from build123d import *

# Parameters (mm, degrees)
SKETCH1_R               = 129.43
BOSS_EXTRUDE1_DEPTH     = 3
CUT_EXTRUDE2_START      = -3
CUT_EXTRUDE2_DEPTH      = 4
CIRPATTERN1_COUNT       = 8
SKETCH4_R               = 3.5
SKETCH4_W               = 25
SKETCH4_H               = 25
CUT_EXTRUDE3_DEPTH      = 3
CUT_EXTRUDE4_DEPTH      = 10
CUT_EXTRUDE5_DEPTH      = 1
CUT_EXTRUDE5_DEPTH_BACK = 3
CUT_EXTRUDE6_DEPTH      = 1
CUT_EXTRUDE6_DEPTH_BACK = 3


with BuildPart() as part:
    # Sketch1 → Boss-Extrude1 (new body)
    with BuildSketch(Plane(origin=(0, 0, 0), x_dir=(1, 0, 0), z_dir=(0, 1, 0))):
        Circle(SKETCH1_R)
    extrude(amount=BOSS_EXTRUDE1_DEPTH)

    # Sketch2 → Cut-Extrude2 (cut)
    with BuildSketch(Plane(origin=(0, 3, 0), x_dir=(1, 0, 0), z_dir=(0, 1, 0)).offset(CUT_EXTRUDE2_START)):
        Polygon((-1.5, 719.582197244), (-1.5, 129.421307751), (-1.5, 119.421307751), (1.5, 119.421307751), (1.5, 129.421307751), (1.5, 719.582197244), (1.5, 1899.903976231), (-1.5, 1899.903976231), align=None)
    cut_extrude2 = extrude(amount=CUT_EXTRUDE2_DEPTH, mode=Mode.SUBTRACT)

    # CirPattern1: Cut-Extrude2 ×8 about axis
    cirpattern1_axis = Axis((0, 0, 0), (0, -1, 0))
    for i in range(1, CIRPATTERN1_COUNT):
        add(cut_extrude2.rotate(cirpattern1_axis, i * 360 / CIRPATTERN1_COUNT), mode=Mode.SUBTRACT)

    # Sketch4 → Cut-Extrude3 (cut)
    with BuildSketch(Plane(origin=(0, 3, 0), x_dir=(1, 0, 0), z_dir=(0, 1, 0))):
        with Locations((20, 20)):
            Circle(SKETCH4_R)
        with Locations((20, -20)):
            Circle(SKETCH4_R)
        with Locations((-20, -20)):
            Circle(SKETCH4_R)
        with Locations((-20, 20)):
            Circle(SKETCH4_R)
        Rectangle(SKETCH4_W, SKETCH4_H)
    extrude(amount=-CUT_EXTRUDE3_DEPTH, mode=Mode.SUBTRACT)

    # Sketch5 → Cut-Extrude4 (cut)
    with BuildSketch(Plane(origin=(0, 3, 0), x_dir=(1, 0, 0), z_dir=(0, 1, 0))):
        Polygon((-42.767689854, -111.089714666), (-39.996051256, -112.237764963), (-26.219447691, -78.978101793), (-28.991086289, -77.830051496), align=None)
        Polygon((-26.137858269, -117.978016449), (-23.366219671, -119.126066746), (-9.589616106, -85.866403575), (-12.361254704, -84.718353278), align=None)
        Polygon((53.935833667, 67.497598822), (67.712437232, 100.757261992), (64.940798634, 101.905312289), (51.164195069, 68.645649119), align=None)
        Polygon((37.306002081, 74.385900604), (51.082605647, 107.645563775), (48.310967049, 108.793614072), (34.534363484, 75.533950901), align=None)
    extrude(amount=-CUT_EXTRUDE4_DEPTH, mode=Mode.SUBTRACT)

    # Sketch6 → Cut-Extrude5 (cut, two sides)
    with BuildSketch(Plane(origin=(0, 3, 0), x_dir=(1, 0, 0), z_dir=(0, 1, 0))) as cut_extrude5_sk:
        Polygon((264.658286272, 696.415643975), (28.490193223, 126.255430735), (21.127814063, 108.481075117), (30.356179145, 104.658561141), (38.225405343, 123.656553754), (274.393498392, 693.816766994), (592.742329798, 1886.329311701), (583.007117678, 1888.928188682), align=None)
    extrude(amount=CUT_EXTRUDE5_DEPTH, mode=Mode.SUBTRACT)
    extrude(cut_extrude5_sk.sketch, amount=-CUT_EXTRUDE5_DEPTH_BACK, mode=Mode.SUBTRACT)

    # Sketch8 → Cut-Extrude6 (cut, two sides)
    with BuildSketch(Plane(origin=(0, 3, 0), x_dir=(1, 0, 0), z_dir=(0, 1, 0))) as cut_extrude6_sk:
        Polygon((-310.659690478, -692.568815319), (-69.116017705, -109.430804605), (-61.752527909, -91.653767674), (-52.555273509, -95.463395183), (-60.423899034, -114.459937644), (-301.967571807, -697.597948358), (-934.16352501, -1790.255908717), (-942.855643681, -1785.226775678), align=None)
    extrude(amount=CUT_EXTRUDE6_DEPTH, mode=Mode.SUBTRACT)
    extrude(cut_extrude6_sk.sketch, amount=-CUT_EXTRUDE6_DEPTH_BACK, mode=Mode.SUBTRACT)


solid = part.part
Model file for the job. Use its own axes, mm. A direction names the side the tool comes from. Round coordinates to 2 decimals unless told otherwise and drop trailing zeros. Loops run counter-clockwise (first coordinate to the right, second up) from the corner with the lowest first, then second, coordinate; pieces in that order, holes last.
1. Band-saw the part on A-A, the plane z = 5. List the corners of the cut face in (x, y), and give its area (3 significant figures).
Check values:
outline: (-129.33, 0) - (-12.5, 0) - (-12.5, 3) - (-129.33, 3) - close; (12.5, 0) - (129.33, 0) - (129.33, 3) - (12.5, 3) - close
area: 701 mm2
2. Band-saw the part on B-B, the plane x = -20. List the corners of the cut face in (y, z), and give its area (3 significant figures).
Check values:
outline: (0, -127.88) - (3, -127.88) - (3, -23.5) - (0, -23.5) - close; (0, -16.5) - (3, -16.5) - (3, 16.5) - (0, 16.5) - close; (0, 23.5) - (3, 23.5) - (3, 103.16) - (0, 103.16) - close; (0, 111) - (3, 111) - (3, 127.88) - (0, 127.88) - close
area: 702 mm2
3. Band-saw the part on C-C, the plane y = 2.45. Count the separate pieces of the cut face and the enclosed holes in it, and give its area (3 significant figures).
Check values:
separate pieces: 1
enclosed holes: 9
area: 50,800 mm2
4. Mould opens along Z. For faces 4 (the cylindrical face through (-32.269, 1.479, 125.343)), 5 (the flat face through (41.52, 1.52, -92.4)), 6 (the flat face through (-2, 3, 27)) say: +Z half, -Z half, draft (parallel to the pull), parting line (faces both ways), or undercut.
Check values:
face 4: +Z half
face 5: undercut
face 6: draft
5. Wall check: probe 1 along Z at (x, y) = (20, 1.35); probe 2 along Z at (x, y) = (2, 2.15). Give the ranges that are in metal, low to high.
Check values:
probe 1: z = -127.88 to -23.5, -16.5 to 16.5, 23.5 to 127.88
probe 2: z = -129.41 to -12.5, 12.5 to 129.41
6. Drop flat-ended pins along their axis: P1, Ø1, axis at y = 1.5, z = 16, coming from the +X side; P2, Ø0.9, axis at x = -0.5, y = 2, coming from the +Z side. Give the stop position or say it passes through.
Check values:
P1: stops at x = 128.5
P2: stops at z = 119.42
7. Tool access for faces 1 (the flat face through (-86.97, 1.48, 89.09)), 2 (the flat face through (-2, 0, 27)), 3 (the flat face through (34.236, 1.521, -114.025)): list every direction of +Z, -Z, +X, -X, +Y, -Y with a clear straight run to the whole face (end or side of a thin tool).
Check values:
face 1: +Y, -Y
face 2: +Z, -Z, +X, -X, -Y
face 3: -Z, +Y, -Y
8. Band-saw the part on D-D, the plane z = -113. List the corners of the cut face in (x, y), and give its area (3 significant figures).
Check values:
outline: (-63.11, 0) - (23, 0) - (23, 3) - (-63.11, 3) - close; (33.81, 0) - (63.11, 0) - (63.11, 3) - (33.81, 3) - close
area: 346 mm2
